Part model, mm, in its own coordinate system. A direction names the side the tool comes from. Round coordinates to 2 decimals unless told otherwise and drop trailing zeros. Order: outer loops, then holes, each group sorted by start corner. A loop starts at its lowest first (then second) coordinate and runs counter-clockwise, first axis right, second up. Notation, with made-up numbers: (5.25, 48.25) - (36.25, 48.25) arc R13 cw to (36.25, 54.25) - close; hole circle Ø6 at (78.25, 47.25). An arc over 180 degrees is marked (long way). Return JSON: item names as keys, results as strings. Group by question number.
Item 1: Probe probe 1 along X at (y, z) = (9.75, 183). List the from-to ranges inside material, lowest first.
Item 2: Drop a flat-ended pin along its axis: pin 1 (5 mm diameter, centred on y = 5.5, z = 423, fed in from -X). Give the stop position or say it passes through.
Item 3: Two-plate mould, pull along X, no slides. Class faces 3 (the face through (0, 10, 345)), 4 (the face through (10, 20, 345)), 5 (the face through (18, 10, 345)), 6 (the face through (10, 2, 345)): released by +X, released by -X, zero draft, split by the parting line, or undercut.
Item 4: Saw through at A-A on z = 59. List the corners of the cut face in (x, y).
Item 5: Tool access for faces 1 (the face through (1, 10, 0)), 2 (the face through (2, 10, 345)): list every direction of +Z, -Z, +X, -X, +Y, -Y with a clear straight run to the whole face (end or side of a thin tool).
```python
from build123d import *

# Parameters (mm, degrees)
SKETCH_1_W          = 20
SKETCH_1_H          = 20
SKETCH_1_W_2        = 16
SKETCH_1_H_2        = 16
EXTRUDE_1_DEPTH     = 700
SKETCH_3_R          = 2
CUT_EXTRUDE_2_DEPTH = 701.571195525
SKETCH_4_R          = 1.5
CUT_EXTRUDE_3_DEPTH = 701.571195525
SKETCH_5_R          = 2.1
CUT_EXTRUDE_4_DEPTH = 701.571195525


with BuildPart() as part:
    # 草图1 → 拉伸-薄壁1 (new body)
    with BuildSketch(Plane.XY):
        with Locations((10, 10)):
            Rectangle(SKETCH_1_W, SKETCH_1_H)
        with Locations((10, 10)):
            Rectangle(SKETCH_1_W_2, SKETCH_1_H_2, mode=Mode.SUBTRACT)
    extrude(amount=EXTRUDE_1_DEPTH)

    # 草图3 → 切除-拉伸2 (cut, through all)
    with BuildSketch(Plane.XZ):
        with Locations(Location((10, 10, 0), (0, 0, 270))):
            Circle(SKETCH_3_R)
        with Locations(Location((10, 30, 0), (0, 0, 270))):
            Circle(SKETCH_3_R)
        with Locations(Location((10, 50, 0), (0, 0, 270))):
            Circle(SKETCH_3_R)
        with Locations(Location((10, 690, 0), (0, 0, 270))):
            Circle(SKETCH_3_R)
        with Locations(Location((10, 670, 0), (0, 0, 270))):
            Circle(SKETCH_3_R)
        with Locations(Location((10, 650, 0), (0, 0, 270))):
            Circle(SKETCH_3_R)
    extrude(amount=-CUT_EXTRUDE_2_DEPTH, mode=Mode.SUBTRACT)

    # 草图4 → 切除-拉伸3 (cut, through all)
    with BuildSketch(Plane.XZ):
        with Locations(Location((10, 170, 0), (0, 0, 270))):
            Circle(SKETCH_4_R)
        with Locations(Location((10, 190, 0), (0, 0, 270))):
            Circle(SKETCH_4_R)
        with Locations(Location((10, 210, 0), (0, 0, 270))):
            Circle(SKETCH_4_R)
        with Locations(Location((10, 490, 0), (0, 0, 270))):
            Circle(SKETCH_4_R)
        with Locations(Location((10, 510, 0), (0, 0, 270))):
            Circle(SKETCH_4_R)
        with Locations(Location((10, 530, 0), (0, 0, 270))):
            Circle(SKETCH_4_R)
        with Locations(Location((10, 473, 0), (0, 0, 270))):
            Circle(SKETCH_4_R)
        with Locations(Location((10, 456, 0), (0, 0, 270))):
            Circle(SKETCH_4_R)
        with Locations(Location((10, 227, 0), (0, 0, 270))):
            Circle(SKETCH_4_R)
        with Locations(Location((10, 244, 0), (0, 0, 270))):
            Circle(SKETCH_4_R)
    extrude(amount=-CUT_EXTRUDE_3_DEPTH, mode=Mode.SUBTRACT)

    # 草图5 → 切除-拉伸4 (cut, through all)
    with BuildSketch(Plane(origin=(20, 0, 0), x_dir=(0, 0, -1), z_dir=(1, 0, 0))):
        with Locations((-70, 10)):
            Circle(SKETCH_5_R)
        with Locations((-110, 10)):
            Circle(SKETCH_5_R)
        with Locations((-150, 10)):
            Circle(SKETCH_5_R)
        with Locations(Location((-550, 10, 0), (0, 0, 180))):
            Circle(SKETCH_5_R)
        with Locations(Location((-590, 10, 0), (0, 0, 180))):
            Circle(SKETCH_5_R)
        with Locations(Location((-630, 10, 0), (0, 0, 180))):
            Circle(SKETCH_5_R)
    extrude(amount=-CUT_EXTRUDE_4_DEPTH, mode=Mode.SUBTRACT)


solid = part.part
```
Filled in:
{
 "1": {"probe 1": "x = 0 to 2, 18 to 20"},
 "2": {"pin 1": "stops at x = 0"},
 "3": {"face 3": "released by -X", "face 4": "zero draft", "face 5": "undercut", "face 6": "undercut"},
 "4": {"outline": "(0, 0) - (20, 0) - (20, 20) - (0, 20) - close; hole (2, 2) - (18, 2) - (18, 18) - (2, 18) - close"},
 "5": {"face 1": "-Z, +X, -X, +Y, -Y", "face 2": "+Z, -Z"}
}
